from build123d import *

# Parameters (mm, degrees)
F0_R     = 254
F1_DEPTH = 88.9
F2_R     = 101.6
F3_DEPTH = 25.4
F4_R     = 101.6
F5_DEPTH = 25.4
F6_R     = 12.7
F7_DEPTH = 127
F8_R     = 12.7
F9_DEPTH = 177.8
F10_R    = 25.4


with BuildPart() as f1:
    # F0 (on Front) → F1 (new body, symmetric)
    with BuildSketch(Plane.XZ):
        Circle(F0_R)
    extrude(amount=F1_DEPTH, both=True)

    # F2 (on face) → F3 (cut)
    with BuildSketch(Plane(origin=(0, 88.9, 0), x_dir=(-1, 0, 0), z_dir=(0, 1, 0))):
        Circle(F2_R)
    extrude(amount=-F3_DEPTH, mode=Mode.SUBTRACT)

    # F4 (on face) → F5 (cut)
    with BuildSketch(Plane.XZ.offset(88.9)):
        Circle(F4_R)
    extrude(amount=-F5_DEPTH, mode=Mode.SUBTRACT)

    # F6 (on face) → F7 (cut)
    with BuildSketch(Plane(origin=(0, 63.5, 0), x_dir=(-1, 0, 0), z_dir=(0, 1, 0))):
        Circle(F6_R)
    extrude(amount=-F7_DEPTH, mode=Mode.SUBTRACT)

    # F8 (on face) → F9 (cut, symmetric)
    with BuildSketch(Plane(origin=(0, 88.9, 0), x_dir=(-1, 0, 0), z_dir=(0, 1, 0))):
        Circle(F8_R)
    extrude(amount=F9_DEPTH, both=True, mode=Mode.SUBTRACT)

    # F10
    f10_edges = [f1.edges().sort_by_distance(p)[0] for p in [
        (-254, -88.9, 0),
        (-254, 88.9, 0),
    ]]
    fillet(f10_edges, radius=F10_R)


solid = f1.part
Can you work these out from the model? Positions are in its coordinate system, mm. A direction names the side the tool comes from. Coordinates: 2 decimals unless noted, no trailing zeros. Write each loop counter-clockwise with the first axis right and the second up, starting at its lowest first coordinate (ties: lowest second). Pieces come first, ordered by that corner, then holes. Notation, with made-up numbers: (52, 42.5) -> (88, 42.5) arc R11 cw to (88, 48.5) -> close; hole circle Ø8 at (85, 70). An arc over 180 degrees is marked (long way). Write item = value, one per line.
(1) On a 3-axis mill with a long thin cutter (end or side, diameter ignored), from which of +Z, -Z, +X, -X, +Y, -Y can I reach the whole of each face in a straight line? I mean faces 4 (the face through (2.75, 0.89, -12.4)), 5 (the face through (21, -63.5, 1)), 6 (the face through (-21, 63.5, 1)). Say none if no direction works.
Verdict:
face_4 = +Y, -Y
face_5 = -Y
face_6 = +Y
(2) Imagine slicing it at A-A (x = 0). Please give me the cut outline in (y, z), and give its area (3 significant figures).
Verdict:
outline = (-88.9, -228.6) arc R25.4 ccw to (-63.5, -254) -> (63.5, -254) arc R25.4 ccw to (88.9, -228.6) -> (88.9, -101.6) -> (63.5, -101.6) -> (63.5, -12.7) -> (-63.5, -12.7) -> (-63.5, -101.6) -> (-88.9, -101.6) -> close; (-88.9, 101.6) -> (-63.5, 101.6) -> (-63.5, 12.7) -> (63.5, 12.7) -> (63.5, 101.6) -> (88.9, 101.6) -> (88.9, 228.6) arc R25.4 ccw to (63.5, 254) -> (-63.5, 254) arc R25.4 ccw to (-88.9, 228.6) -> close
area = 76,200 mm^2
(3) If I drill on probe 1 along Z at (x, y) = (0, 19); probe 2 along X at (y, z) = (3, 8); probe 3 along Z at (x, y) = (0, -80.5), over which ranges is the centre line in solid material (lowest first)?
Verdict:
probe_1 = -254 to -12.7, 12.7 to 254
probe_2 = -253.87 to -9.86, 9.86 to 253.87
probe_3 = -247.47 to -101.6, 101.6 to 247.47
(4) Imagine slicing it at C-C (y = 14.5). Please give me the cut outline in (x, z), and give its area (3 significant figures).
Verdict:
outline = circle Ø508 at (0, 0); hole circle Ø25.4 at (0, 0)
area = 202,000 mm^2
(5) Imagine slicing it at B-B (z = 0). Please give me the cut outline in (x, y), and give its area (3 significant figures).
Verdict:
outline = (-254, -63.5) arc R25.4 ccw to (-228.6, -88.9) -> (-101.6, -88.9) -> (-101.6, -63.5) -> (-12.7, -63.5) -> (-12.7, 63.5) -> (-101.6, 63.5) -> (-101.6, 88.9) -> (-228.6, 88.9) arc R25.4 ccw to (-254, 63.5) -> close; (12.7, -63.5) -> (101.6, -63.5) -> (101.6, -88.9) -> (228.6, -88.9) arc R25.4 ccw to (254, -63.5) -> (254, 63.5) arc R25.4 ccw to (228.6, 88.9) -> (101.6, 88.9) -> (101.6, 63.5) -> (12.7, 63.5) -> close
area = 76,200 mm^2
(6) Thinking about a two-plate mould opening in X: for faces 1 (the face through (-55.06, -0.89, -247.96)), 2 (the face through (98, 88.9, -48)), 3 (the face through (22.025, 76.378, -99.184)), which applies, +X half, -X half, draft (parallel to the pull), parting line (faces both ways), or undercut?
Verdict:
face_1 = parting line
face_2 = draft
face_3 = undercut
(7) For pin 1 (2 mm diameter, centred on x = -199.5, z = -129, fed in from +Y); pin 2 (12 mm diameter, centred on x = -192.5, y = -19, fed in from +Z); pin 3 (4 mm diameter, centred on x = 110.5, y = -51, fed in from +Z); pin 4 (23 mm diameter, centred on x = 0, z = 0, fed in from +Y), each with a flat end and sliding along its axis, tell me the tip position at first contact or that it passes through.
Verdict:
pin_1 = 87.62
pin_2 = 172.43
pin_3 = 229.66
pin_4 = through
